from build123d import *

# Parameters (mm, degrees)
CYLINDER001_R     = 4.05
CYLINDER001_DEPTH = 28
CYLINDER_R        = 6
CYLINDER_DEPTH    = 5
SKETCH_R          = 7
PAD_DEPTH         = 2
CHAMFER_SIZE      = 0.99
CHAMFER001_SIZE   = 1
CHAMFER002_SIZE   = 0.5


with BuildPart() as cilindro001:
    # Cylinder001 → Cylinder001 (new body)
    with BuildSketch(Plane.XY.offset(-1)):
        Circle(CYLINDER001_R)
    extrude(amount=CYLINDER001_DEPTH)


with BuildPart() as chamfer002:
    # Cylinder → Cylinder (new body)
    with BuildSketch(Plane.XY):
        Circle(CYLINDER_R)
    extrude(amount=CYLINDER_DEPTH)

    # Sketch → Pad (new body)
    with BuildSketch(Plane.XY.offset(5)):
        Circle(SKETCH_R)
    extrude(amount=PAD_DEPTH)

    # Cut: cut Cilindro001
    add(cilindro001.part, mode=Mode.SUBTRACT)

    # Chamfer
    chamfer_edges = [chamfer002.edges().sort_by_distance(p)[0] for p in [
        (-6, 0, 5),
    ]]
    chamfer(chamfer_edges, length=CHAMFER_SIZE)

    # Chamfer001
    chamfer001_edges = [chamfer002.edges().sort_by_distance(p)[0] for p in [
        (-6, 0, 0),
    ]]
    chamfer(chamfer001_edges, length=CHAMFER001_SIZE)

    # Chamfer002
    chamfer002_edges = [chamfer002.edges().sort_by_distance(p)[0] for p in [
        (-4.05, 0, 7),
    ]]
    chamfer(chamfer002_edges, length=CHAMFER002_SIZE)


solid = chamfer002.part
Geometry check sheet. Reference: the model listing, model coordinates, mm. Give positions to 0.01 mm unless a question says otherwise; leave off trailing zeros. Order: outer loops, then holes, each group sorted by start corner. A loop starts at its lowest first (then second) coordinate and runs counter-clockwise, first axis right, second up. Notation, with made-up numbers: (46.25, 10) - (94.25, 10) arc R32 ccw to (94.25, 49) - close; hole circle Ø9 at (70, 51.25). An arc over 180 degrees is marked (long way). Answer as a JSON object with one key per item and string values.
(1) Draft check along X on faces 1 (the cylindrical face through (-6, 0, 2)), 2 (the cylindrical face through (-0.878, -3.954, 3.204)), 3 (the flat face through (2, -4, 0)). Enter one of: released by +X, released by -X, zero draft, split by the parting line, or undercut.
Report:
{"face 1": "split by the parting line", "face 2": "undercut", "face 3": "zero draft"}
(2) Cross-section at C-C (z = 5.75). Record the cut outline in (x, y), then the cut area to 3 significant figures.
Report:
{"outline": "circle Ø14 at (0, 0); hole circle Ø8.1 at (0, 0)", "area": "102 mm^2"}
(3) Material ranges on line 1 (Y direction, x = 0, z = 3.25); line 2 (Y direction, x = -1.75, z = 6); line 3 (X direction, y = -2, z = 2), recorded low to high.
Report:
{"line 1": "-6 to -4.05, 4.05 to 6", "line 2": "-6.78 to -3.65, 3.65 to 6.78", "line 3": "-5.66 to -3.52, 3.52 to 5.66"}
(4) Depth check by flat-ended pin: pin 1 Ø6.5 at (x, y) = (0, 0) entering from +Z; pin 2 Ø1.5 at (x, z) = (5, 3.5) entering from +Y. Enter the tip coordinate at first touch or a pass-through.
Report:
{"pin 1": "through", "pin 2": "y = 4.24"}
